Input: part model. Units: mm. Frame: model coordinates. A direction names the side the tool comes from. Round coordinates to 2 decimals unless told otherwise and drop trailing zeros. Order: outer loops, then holes, each group sorted by start corner. A loop starts at its lowest first (then second) coordinate and runs counter-clockwise, first axis right, second up. Notation, with made-up numbers: (43, 51) -> (70, 51) arc R28 ccw to (70, 90) -> close; hole circle Ø1 at (73, -14.5). An arc over 180 degrees is marked (long way). Use a Markdown table: item, result.
Autodesk Inventor part; units mm, degrees
ref_plane "YZ Plane" through (0, 0, 0) normal (1, 0, 0) x (0, 1, 0)
ref_plane "XZ Plane" through (0, 0, 0) normal (0, 1, 0) x (-1, 0, 0)
ref_plane "XY Plane" through (0, 0, 0) normal (0, 0, 1) x (1, 0, 0)
sketch "Esquisse1" plane through (0, 0, 0) normal (0, 0, 1) x (1, 0, 0)
  line L0 (110, -100) -> (-110, -100)
  line L1 (-170, -60) -> (-170, 60)
  line L2 (170, 60) -> (170, -60)
  line L3 (170, -100) -> (-170, 100) construction
  line L4 (-170, -100) -> (170, 100) construction
  line L5 (-90, 100) -> (-170, 60)
  line L6 (90, 100) -> (170, 60)
  line L7 (-170, -60) -> (-110, -100)
  line L8 (110, -100) -> (170, -60)
  line L9 (-90, 100) -> (90, 100)
  point P0 (0, 0)
  point P1 (0, 0)
  dimension "d0" = 340
  dimension "d1" = 80
  dimension "d2" = 40
  dimension "d3" = 80
  dimension "d4" = 40
  dimension "d5" = 40
  dimension "d6" = 60
  dimension "d7" = 60
  dimension "d8" = 40
  dimension "d17" = 100
extrude "Extrusion1" add sketch "Esquisse1" along normal blind 6
sketch "Esquisse2" plane through (0, 0, 6) normal (0, 0, 1) x (1, 0, 0)
  line L0 (-54, 90) -> (54, 90)
  line L1 (-156, 0) -> (156, 0)
  line L2 (-170, 60) -> (-170, -60)
  line L3 (170, -60) -> (170, 60)
  line L4 (-110, -100) -> (110, -100)
  line L5 (90, 100) -> (-69, 100)
  line L6 (-156, 0) -> (-156, 51.3475)
  line L7 (-156, 0) -> (-156, -52.5074)
  line L8 (156, 0) -> (156, 51.3475)
  line L9 (156, 0) -> (156, -52.5074)
  line L10 (170, 60) -> (90, 100)
  line L11 (110, -100) -> (170, -60)
  line L12 (-170, -60) -> (-110, -100)
  line L13 (-90, 100) -> (-170, 60)
  line L14 (90, 100) -> (-90, 100)
  point P0 (0, 0)
  point P1 (0, 0)
  point P2 (-54, -90)
  point P3 (54, -90)
  point P4 (0, 0)
  dimension "d21" = 14
  dimension "d22" = 14
  dimension "d23" = 10
  dimension "d24" = 108
  dimension "d25" = 54
  dimension "d29" = 108
  dimension "d30" = 10
  dimension "d31" = 10
  dimension "d32" = 56
  dimension "d34" = 56
  dimension "d42" = 14
  dimension "d43" = 14
  dimension "d44" = 14
  dimension "d45" = 14
hole "Perçage1" at (-156, -52.5074, 6) at (-156, 51.3475, 6) at (-54, 90, 6) at (54, 90, 6) at (156, 51.3475, 6) at (156, -52.5074, 6) at (54, -90, 6) at (-54, -90, 6) direction (0, 0, -1) diameter 8 end through all
sketch "Esquisse3" plane through (0, 0, 6) normal (0, 0, 1) x (1, 0, 0)
  line L0 (-6, 84) -> (6, 84)
  line L1 (6, 84) -> (6, 76)
  line L2 (6, 76) -> (-6, 76)
  line L3 (-6, 76) -> (-6, 84)
  line L4 (-121.0377, 66.5926) -> (-110.3046, 71.9592)
  line L5 (-110.3046, 71.9592) -> (-106.7269, 64.8037)
  line L6 (-106.7269, 64.8037) -> (-117.46, 59.4372)
  line L7 (-117.46, 59.4372) -> (-121.0377, 66.5926)
  line L8 (-113.9841, -76.4747) -> (-102.7209, -80.6148)
  line L9 (-102.7209, -80.6148) -> (-99.9608, -73.106)
  line L10 (-99.9608, -73.106) -> (-111.2241, -68.9659)
  line L11 (-111.2241, -68.9659) -> (-113.9841, -76.4747)
  line L12 (-90, 100) -> (-170, 60)
  circle A0 centre (-156, 51.3475) radius 4
  circle A1 centre (-156, -52.5074) radius 4
  circle A2 centre (-54, -90) radius 4
  line L13 (-156, -52.5074) -> (-54, -90)
  line L14 (0, 0) -> (0, -39.4059)
  line L15 (0, 0) -> (52.1624, 0)
  line L16 (121.0377, 66.5926) -> (110.3046, 71.9592)
  line L17 (110.3046, 71.9592) -> (106.7269, 64.8037)
  line L18 (106.7269, 64.8037) -> (117.46, 59.4372)
  line L19 (117.46, 59.4372) -> (121.0377, 66.5926)
  line L20 (113.9841, -76.4747) -> (102.7209, -80.6148)
  line L21 (102.7209, -80.6148) -> (99.9608, -73.106)
  line L22 (99.9608, -73.106) -> (111.2241, -68.9659)
  line L23 (111.2241, -68.9659) -> (113.9841, -76.4747)
  line L24 (156, -52.5074) -> (54, -90)
  line L25 (90, 100) -> (-90, 100)
  line L26 (-6, -84) -> (6, -84)
  line L27 (6, -84) -> (6, -76)
  line L28 (6, -76) -> (-6, -76)
  line L29 (-6, -76) -> (-6, -84)
  dimension "d46" = 16
  dimension "d47" = 24
  dimension "d48" = 12
  dimension "d49" = 38.089
  dimension "d52" = 8
  dimension "d53" = 12
  dimension "d54" = 47.705
  dimension "d55" = 12
  dimension "d56" = 8
  dimension "d57" = 6
  dimension "d58" = 16
extrude "Extrusion2" cut sketch "Esquisse3" against normal blind 10 contours L0 L1 L2 L3 | L4 L5 L6 L7 | L11 L10 L9 L8 | L19 L18 L17 L16 | L20 L21 L22 L23 | L29 L28 L27 L26
sketch "Esquisse4" plane through (0, 0, 6) normal (0, 0, 1) x (1, 0, 0)
  line L0 (0, 0) -> (0, 42.3404)
  line L1 (-152, 25) -> (-158, 25)
  line L2 (-160, 23) -> (-160, -23)
  line L3 (-158, -25) -> (-152, -25)
  line L4 (-150, -23) -> (-150, 23)
  line L5 (-158, 25) -> (-160, 23)
  line L6 (-152, 25) -> (-150, 23)
  line L7 (-152, -25) -> (-150, -23)
  line L8 (-160, -23) -> (-158, -25)
  line L9 (152, 25) -> (158, 25)
  line L10 (160, 23) -> (160, -23)
  line L11 (158, -25) -> (152, -25)
  line L12 (150, -23) -> (150, 23)
  line L13 (158, 25) -> (160, 23)
  line L14 (152, 25) -> (150, 23)
  line L15 (152, -25) -> (150, -23)
  line L16 (160, -23) -> (158, -25)
  point P0 (-150, 25)
  point P1 (-160, -25)
  point P2 (-160, 25)
  point P3 (-150, -25)
  point P4 (150, 25)
  point P5 (160, -25)
  point P6 (160, 25)
  point P7 (150, -25)
  dimension "d59" = 10
  dimension "d60" = 150
  dimension "d61" = 50
  dimension "d62" = 25
  dimension "d63" = 2
  dimension "d64" = 2
  dimension "d65" = 2
  dimension "d66" = 2
  dimension "d67" = 2
  dimension "d68" = 2
  dimension "d69" = 2
  dimension "d70" = 2
extrude "Extrusion3" cut sketch "Esquisse4" against normal blind 10
properties part number "Support_Carte"
1) Contact query for flat-ended pins moving along their axis: P1, Ø7, axis at x = 54, y = 90, coming from the +Z side; P2, Ø3, axis at x = -155, z = 2.5, coming from the +Y side; P3, Ø3, axis at y = 80.5, z = 2, coming from the +X side; P4, Ø8, axis at x = -102.5, y = 34, coming from the -Z side. Output: stop coordinate, or through.
Answer key:
| item | result |
|---|---|
| P1 | passes through |
| P2 | stops at y = 68.25 |
| P3 | stops at x = 132 |
| P4 | stops at z = 0 |
2) Set-up query: faces 1 (the face through (-2, 1, 0)), 2 (the face through (108.431, -78.516, 3.042)). Return all of +Z, -Z, +X, -X, +Y, -Y with unobstructed straight access to the full face (end or side cutting, diameter ignored); none if empty.
Answer key:
| item | result |
|---|---|
| face 1 | -Z, +X, -X, +Y, -Y |
| face 2 | +Z, -Z |
3) Cut plane C-C on z = 4.55. State how many separate pieces and enclosed holes the cut face has, and give its area (3 significant figures).
Answer key:
| item | result |
|---|---|
| separate pieces | 1 |
| enclosed holes | 16 |
| area | 60,400 mm^2 |
4) Cut plane B-B on x = 2. Return loops of the section in (y, z), and give its area (3 significant figures).
Answer key:
| item | result |
|---|---|
| outline | (-100, 0) -> (-84, 0) -> (-84, 6) -> (-100, 6) -> close; (-76, 0) -> (76, 0) -> (76, 6) -> (-76, 6) -> close; (84, 0) -> (100, 0) -> (100, 6) -> (84, 6) -> close |
| area | 1,100 mm^2 |
5) Cut plane A-A on y = -90. Return loops of the section in (x, z), and give its area (3 significant figures).
Answer key:
| item | result |
|---|---|
| outline | (-125, 0) -> (-58, 0) -> (-58, 6) -> (-125, 6) -> close; (-50, 0) -> (50, 0) -> (50, 6) -> (-50, 6) -> close; (58, 0) -> (125, 0) -> (125, 6) -> (58, 6) -> close |
| area | 1,400 mm^2 |
6) Ray query, probe 1 along Y at (x, z) = (54, 3.15); probe 2 along X at (y, z) = (1.5, 4.6); probe 3 along X at (y, z) = (-87, 2.05). Return the intervals inside material, ascending.
Answer key:
| item | result |
|---|---|
| probe 1 | y = -100 to -94, -86 to 86, 94 to 100 |
| probe 2 | x = -170 to -160, -150 to 150, 160 to 170 |
| probe 3 | x = -129.5 to -56.65, -51.35 to 51.35, 56.65 to 129.5 |
